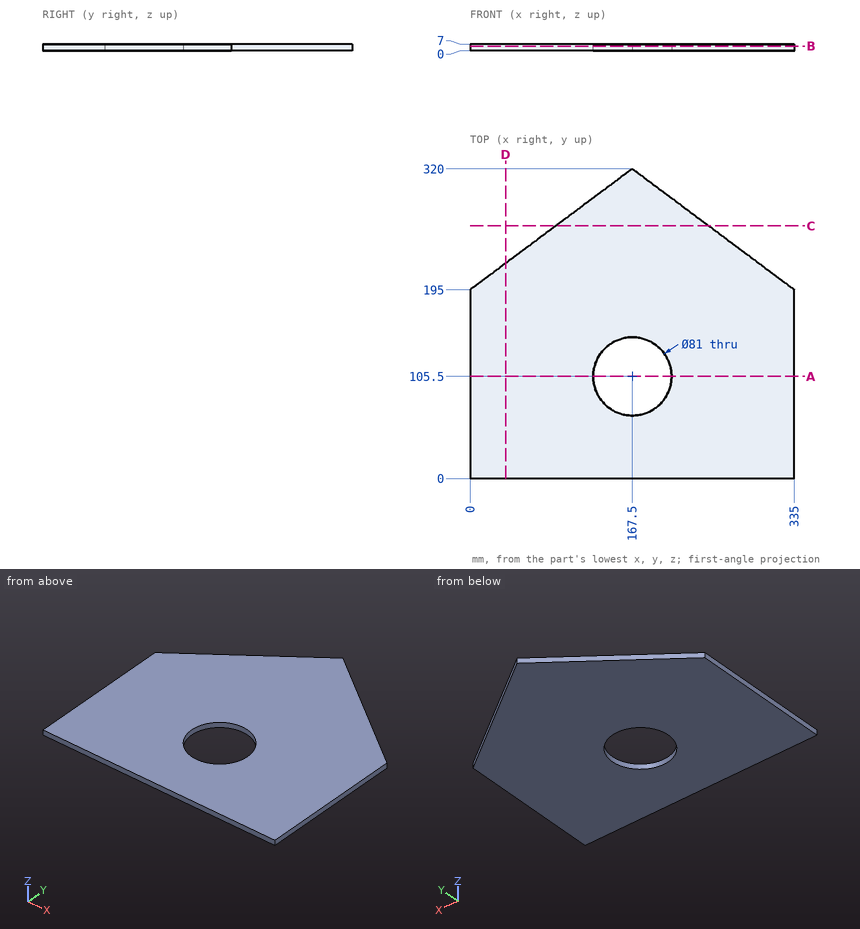
Geometry: see drawing. Coordinates: mm, zero at the bounding-box minimum. Give positions to 0.01 mm unless a question says otherwise; leave off trailing zeros. Loops run counter-clockwise (first coordinate to the right, second up) from the corner with the lowest first, then second, coordinate; pieces in that order, holes last. Notation, with made-up numbers: (66, -29) -> (112, -29) arc R23 ccw to (112, -9) -> close; hole circle Ø11 at (-29.75, -1.5). An arc over 180 degrees is marked (long way). Use CSV: the item, a comma, the result in double quotes.
(1) Cut plane B-B (z = 4.75). Output: boundary loops of the cut face in (x, y).
From the geometry:
outline,"(0, 0) -> (335, 0) -> (335, 195) -> (167.5, 320) -> (0, 195) -> close; hole circle Ø81 at (167.5, 105.5)"
(2) Cut plane C-C (y = 261). Output: boundary loops of the cut face in (x, z), plus the area to 3 significant figures.
From the geometry:
outline,"(88.44, 0) -> (246.56, 0) -> (246.56, 7) -> (88.44, 7) -> close"
area,"1,110 mm^2"
(3) Cut plane A-A (y = 105.5). Output: boundary loops of the cut face in (x, z).
From the geometry:
outline,"(0, 0) -> (127, 0) -> (127, 7) -> (0, 7) -> close; (208, 0) -> (335, 0) -> (335, 7) -> (208, 7) -> close"
(4) Ray query, line 1 along X through (y, z) = (105.5, 5.25); line 2 along Y through (x, z) = (167.5, 3.75); line 3 along Y through (x, z) = (187, 6). Return the intervals inside material, ascending. Write a range as [from, to].
From the geometry:
line 1,"[0, 127], [208, 335]"
line 2,"[0, 65], [146, 320]"
line 3,"[0, 70], [141, 305.45]"
(5) Cut plane D-D (x = 36.5). Output: boundary loops of the cut face in (y, z), plus the area to 3 significant figures.
From the geometry:
outline,"(0, 0) -> (222.24, 0) -> (222.24, 7) -> (0, 7) -> close"
area,"1,560 mm^2"
(6) First-contact query: P1, Ø1.5, axis at y = 205, z = 5.5, coming from the +X side (3 decimals). Flat tip, straight axial feed; report the tip coordinate or a pass-through.
From the geometry:
P1,"x = 322.605"
